Read the model definition and answer for the solid it produces. Units are mm, in the model's axes. A direction names the side the tool comes from. Round coordinates to 2 decimals unless told otherwise and drop trailing zeros. Write each loop counter-clockwise with the first axis right and the second up, starting at its lowest first coordinate (ties: lowest second). Pieces come first, ordered by that corner, then holes. Notation, with made-up numbers: (-36, 34) - (-12, 34) arc R16 cw to (-12, 65) - close; hole circle Ø1 at (63, -10). An arc over 180 degrees is marked (long way). One line per item, written item: value. Start each with the question number.
(1) Flat-ended cylindrical pins translate along their axes: pin 1 Ø2 at (x, z) = (0, -25.29) entering from -Y; pin 2 Ø3 at (y, z) = (-1.5, 24) entering from -X; pin 3 Ø3 at (y, z) = (2, 27.5) entering from -X; pin 4 Ø1.5 at (y, z) = (3, 40.5) entering from -X. Find the tip coordinate at first contact, or state that the pin passes through.
(2) Find the intervals of material crossed by L1, parallel to Z at x = 0, y = -5.15; L2, parallel to X at y = 0, z = -22; L3, parallel to Z at x = 0, y = -4, in increasing order.
(3) A cutting plane is placed at B-B, the plane y = 0. Determine the outline of the cut face in (x, z), plus the area to 3 significant figures.
(4) A cutting plane is placed at C-C, the plane z = 90. Determine the outline of the cut face in (x, y).
(5) The mould has two halves that part along Y. Classify faces 5 (the face through (0, 0, -18.066)), 6 (the face through (1, -5, -7.112)), 7 (the face through (-1.38, 6.2, -19.99)): +Y half, -Y half, draft (parallel to the pull), parting line (faces both ways), or undercut.
(6) A cutting plane is placed at A-A, the plane x = 0. Determine the outline of the cut face in (y, z).
(7) For faces 1 (the face through (3, 1, -32.512)), 2 (the face through (-0.65, 2.93, -25.39)), 3 (the face through (-0.28, 2.134, 62.611)), 4 (the face through (-1.4, -4.4, -26.3)), determine the directions among +Z, -Z, +X, -X, +Y, -Y from which every point of the face is accessible in a straight line to the end or side of a thin tool.
from build123d import *

# Parameters (mm, degrees)
F0_R      = 2.15265
F1_DEPTH  = 127
F2_R      = 4.7625
F3_DEPTH  = 7.112
F4_W      = 50.8
F4_H      = 50.8
F5_DEPTH  = 25.4
F6_R      = 3
F7_DEPTH  = 14.44625
F8_R      = 1.7272
F9_DEPTH  = 23.9470875132
F10_W     = 50.8
F10_H     = 50.8
F10_R     = 6.35
F11_DEPTH = 25.4
F12_SIZE  = 0.254


with BuildPart() as f1:
    # F0 (on Top) → F1 (new body)
    with BuildSketch(Plane.XY):
        Circle(F0_R)
    extrude(amount=F1_DEPTH)

    # F2 (on face) → F3 (join)
    with BuildSketch(Plane(origin=(0, 0, 0), x_dir=(1, 0, 0), z_dir=(0, 0, -1))):
        Circle(F2_R)
    extrude(amount=F3_DEPTH)

    # F4 (on face) → F5 (join)
    with BuildSketch(Plane(origin=(0, 0, -7.112), x_dir=(1, 0, 0), z_dir=(0, 0, -1))):
        Rectangle(F4_W, F4_H)
    extrude(amount=F5_DEPTH)

    # F6 (on face) → F7 (cut)
    with BuildSketch(Plane(origin=(0, 0, -32.512), x_dir=(1, 0, 0), z_dir=(0, 0, -1))):
        Circle(F6_R)
    extrude(amount=-F7_DEPTH, mode=Mode.SUBTRACT)

    # F8 (on face) → F9 (cut, up to face)
    with BuildSketch(Plane.XZ.offset(25.4)):
        with Locations((0, -25.288875)):
            Circle(F8_R)
    extrude(amount=-F9_DEPTH, mode=Mode.SUBTRACT)

    # F10 (on face) → F11 (cut, through all)
    with BuildSketch(Plane(origin=(0, 0, -32.512), x_dir=(1, 0, 0), z_dir=(0, 0, -1))):
        Rectangle(F10_W, F10_H)
        Circle(F10_R, mode=Mode.SUBTRACT)
    extrude(amount=-F11_DEPTH, mode=Mode.SUBTRACT)

    # F12
    f12_edges = [f1.edges().sort_by_distance(p)[0] for p in [
        (-4.7625, 0, 0),
    ]]
    chamfer(f12_edges, length=F12_SIZE)


solid = f1.part
Here are the results:
1. pin 1: y = 2.83
1. pin 2: x = -2.15
1. pin 3: x = -2.09
1. pin 4: through
2. L1: -32.51 to -27.02, -23.56 to -7.11
2. L2: -6.35 to -3, 3 to 6.35
2. L3: -32.51 to -27.02, -23.56 to 0
3. outline: (-6.35, -32.51) - (-3, -32.51) - (-3, -18.07) - (3, -18.07) - (3, -32.51) - (6.35, -32.51) - (6.35, -7.11) - (4.76, -7.11) - (4.76, -0.25) - (4.51, 0) - (2.15, 0) - (2.15, 127) - (-2.15, 127) - (-2.15, 0) - (-4.51, 0) - (-4.76, -0.25) - (-4.76, -7.11) - (-6.35, -7.11) - close
3. area: 850 mm²
4. outline: circle Ø4.31 at (0, 0)
5. face 5: undercut
5. face 6: draft
5. face 7: parting line
6. outline: (-6.35, -32.51) - (-3, -32.51) - (-3, -27.02) - (-6.35, -27.02) - close; (-6.35, -23.56) - (-3, -23.56) - (-3, -18.07) - (3, -18.07) - (3, -32.51) - (6.35, -32.51) - (6.35, -7.11) - (4.76, -7.11) - (4.76, -0.25) - (4.51, 0) - (2.15, 0) - (2.15, 127) - (-2.15, 127) - (-2.15, 0) - (-4.51, 0) - (-4.76, -0.25) - (-4.76, -7.11) - (-6.35, -7.11) - close
7. face 1: -Z, +X, -X, +Y, -Y
7. face 2: -Z
7. face 3: +Z
7. face 4: -Y
